Part model, mm, in its own coordinate system. A direction names the side the tool comes from. Give positions to 0.01 mm unless a question says otherwise; leave off trailing zeros. Order: outer loops, then holes, each group sorted by start corner. A loop starts at its lowest first (then second) coordinate and runs counter-clockwise, first axis right, second up. Notation, with made-up numbers: (47, 5.5) - (71, 5.5) arc R25 ccw to (71, 29.5) - close; hole circle Ø3 at (34.25, 85.5). An arc over 180 degrees is marked (long way). Use one line per item in the form item = value. Start each with the question number.
1. Band-saw the part on A-A, the plane z = -35.5. List the corners of the cut face in (x, y) (3 decimals), plus the area to 3 significant figures.
2. Band-saw the part on B-B, the plane y = -7. List the corners of the cut face in (x, z) (3 decimals).
3. Pin check, flat tips, straight feed: P1, Ø3, axis at x = 7, z = -28, coming from the -Y side; P2, Ø1.8, axis at x = 10.325, y = -10.25, coming from the -Z side; P3, Ø6, axis at y = 7.5, z = -42.5, coming from the -X side (3 decimals). Stop position of each tip, or through.
4. Drill centre lines: line 1 (Y direction, x = -12, z = -44); line 2 (Y direction, x = -7, z = -17.5); line 3 (Z direction, x = -8.75, y = 11). Where is each one in solid material? Low to high.
5. Tool access for faces 5 (the face through (10.3, -10.2, 6)), 6 (the face through (12.425, 0, 2)), 7 (the face through (-10.617, 11.744, 5.165)), 8 (the face through (14, -13, -48)): list every direction of +Z, -Z, +X, -X, +Y, -Y with a clear straight run to the whole face (end or side of a thin tool).
6. Pull direction Y, two halves, no side cores. Call faces 1 (the face through (14, 7, -49)), 2 (the face through (-10, -3.5, 2)), 3 (the face through (15, -16.5, -9)), 4 (the face through (-6.85, -13.54, 3.77)): +Y half, -Y half, draft (parallel to the pull), parting line (faces both ways), or undercut.
7. Band-saw the part on C-C, the plane y = 15.5. List the corners of the cut face in (x, z) (3 decimals).
from build123d import *

# Parameters (mm, degrees)
SKETCH2_W           = 33.15
SKETCH2_H           = 33
BOSS_EXTRUDE1_DEPTH = 7.5
SKETCH3_R           = 0.762
CUT_EXTRUDE1_DEPTH  = 6
SKETCH4_W           = 5.3
SKETCH4_H           = 7
CUT_EXTRUDE2_DEPTH  = 3.4
SKETCH5_W           = 17.312690108
SKETCH5_H           = 1.808425299
CUT_EXTRUDE3_DEPTH  = 2
SKETCH6_W           = 5.3
SKETCH6_H           = 3.3
CUT_EXTRUDE4_DEPTH  = 25.560753755
CHAMFER3_SIZE       = 11
CHAMFER3_SIZE2      = 5.848803748
BOSS_EXTRUDE2_DEPTH = 52.5
SKETCH8_W           = 33.15
SKETCH8_H           = 60
BOSS_EXTRUDE3_DEPTH = 1
SKETCH9_W           = 3
SKETCH9_H           = 34
CUT_EXTRUDE5_DEPTH  = 60
SKETCH10_R          = 0.762
CUT_EXTRUDE6_DEPTH  = 6
SKETCH11_R          = 0.762
CUT_EXTRUDE7_DEPTH  = 6
SKETCH12_R          = 0.762
CUT_EXTRUDE9_DEPTH  = 7
SKETCH13_W          = 3
SKETCH13_H          = 5
CUT_EXTRUDE10_DEPTH = 1.5
SKETCH14_W          = 52.5
SKETCH14_H          = 1
BOSS_EXTRUDE4_DEPTH = 1
SKETCH15_R          = 0.762
CUT_EXTRUDE11_DEPTH = 3.5


with BuildPart() as part:
    # Sketch2 → Boss-Extrude1 (new body)
    with BuildSketch(Plane.XY):
        Rectangle(SKETCH2_W, SKETCH2_H)
    extrude(amount=BOSS_EXTRUDE1_DEPTH)

    # Sketch3 → Cut-Extrude1 (cut)
    with BuildSketch(Plane.XY):
        with Locations((10.325, 10.25)):
            Circle(SKETCH3_R)
        with Locations((-10.325, 10.25)):
            Circle(SKETCH3_R)
        with Locations((10.325, -10.25)):
            Circle(SKETCH3_R)
        with Locations((-10.325, -10.25)):
            Circle(SKETCH3_R)
    extrude(amount=CUT_EXTRUDE1_DEPTH, mode=Mode.SUBTRACT)

    # Sketch4 → Cut-Extrude2 (cut)
    with BuildSketch(Plane.XY):
        with Locations((9.775, 0)):
            Rectangle(SKETCH4_W, SKETCH4_H)
        with Locations((-9.775, 0)):
            Rectangle(SKETCH4_W, SKETCH4_H)
    extrude(amount=CUT_EXTRUDE2_DEPTH, mode=Mode.SUBTRACT)

    # Sketch5 → Cut-Extrude3 (cut)
    with BuildSketch(Plane.XY):
        with Locations((-0.109621432, -11.80915301)):
            Rectangle(SKETCH5_W, SKETCH5_H)
    extrude(amount=CUT_EXTRUDE3_DEPTH, mode=Mode.SUBTRACT)

    # Sketch6 → Cut-Extrude4 (cut, through all)
    with BuildSketch(Plane.XY):
        Rectangle(SKETCH6_W, SKETCH6_H)
    extrude(amount=CUT_EXTRUDE4_DEPTH, mode=Mode.SUBTRACT)

    # Chamfer3
    chamfer3_edges = [part.edges().sort_by_distance(p)[0] for p in [
        (2.65, 0, 7.5),
        (0, 1.65, 7.5),
        (-2.65, 0, 7.5),
        (0, -1.65, 7.5),
    ]]
    chamfer3_side = [part.faces().sort_by_distance(p)[0] for p in [
        (-16.107247662, 0, 7.5),
    ]]
    chamfer(chamfer3_edges, length=CHAMFER3_SIZE, length2=CHAMFER3_SIZE2, reference=chamfer3_side[0])

    # Sketch7 → Boss-Extrude2 (add)
    with BuildSketch(Plane.XY):
        Polygon((13.575, -16.5), (17.575, -16.5), (17.575, 16.5), (-16.575, 16.5), (-16.575, -16.5), (-13.575, -16.5), (-13.575, 13.5), (13.575, 13.5), align=None)
    extrude(amount=-BOSS_EXTRUDE2_DEPTH)

    # Sketch8 → Boss-Extrude3 (add)
    with BuildSketch(Plane(origin=(0, 16.5, 0), x_dir=(1, 0, 0), z_dir=(0, 1, 0))):
        with Locations((0, 22.5)):
            Rectangle(SKETCH8_W, SKETCH8_H)
    extrude(amount=BOSS_EXTRUDE3_DEPTH)

    # Sketch9 → Cut-Extrude5 (cut)
    with BuildSketch(Plane(origin=(0, 0, -52.5), x_dir=(-1, 0, 0), z_dir=(0, 0, -1))):
        with Locations((15.075, 0.5)):
            Rectangle(SKETCH9_W, SKETCH9_H)
    extrude(amount=-CUT_EXTRUDE5_DEPTH, mode=Mode.SUBTRACT)

    # Sketch10 → Cut-Extrude6 (cut)
    with BuildSketch(Plane.ZY.offset(13.575)):
        with Locations((-44, 15.5)):
            Circle(SKETCH10_R)
        with Locations(Location((5, 11, 0), (0, 0, 180))):
            Circle(SKETCH10_R)
        with Locations((5, -10)):
            Circle(SKETCH10_R)
    extrude(amount=-CUT_EXTRUDE6_DEPTH, mode=Mode.SUBTRACT)

    # Sketch11 → Cut-Extrude7 (cut)
    with BuildSketch(Plane(origin=(0, -16.5, 0), x_dir=(-1, 0, 0), z_dir=(0, -1, 0))):
        with Locations(Location((-15.575, 44, 0), (0, 0, 90))):
            Circle(SKETCH11_R)
        with Locations((-15.575, -51.5)):
            Circle(SKETCH11_R)
        with Locations(Location((7.075, -4.5, 0), (0, 0, 90))):
            Circle(SKETCH11_R)
        with Locations(Location((-11.075, -4.5, 0), (0, 0, 90))):
            Circle(SKETCH11_R)
    extrude(amount=-CUT_EXTRUDE7_DEPTH, mode=Mode.SUBTRACT)

    # Sketch12 → Cut-Extrude9 (cut)
    with BuildSketch(Plane(origin=(0, 0, -52.5), x_dir=(-1, 0, 0), z_dir=(0, 0, -1))):
        with Locations((-15.575, 15.5)):
            Circle(SKETCH12_R)
        with Locations((-15.575, -14.5)):
            Circle(SKETCH12_R)
        with Locations((11.575, 15.5)):
            Circle(SKETCH12_R)
    extrude(amount=-CUT_EXTRUDE9_DEPTH, mode=Mode.SUBTRACT)

    # Sketch13 → Cut-Extrude10 (cut)
    with BuildSketch(Plane.ZY.offset(-13.575)):
        Polygon((-46.5, 7), (-52.5, 7), (-52.5, -13), (-46.5, -13), (-46.5, -8), align=None)
        with Locations((-45, -10.5)):
            Rectangle(SKETCH13_W, SKETCH13_H)
    extrude(amount=-CUT_EXTRUDE10_DEPTH, mode=Mode.SUBTRACT)

    # Sketch14 → Boss-Extrude4 (add)
    with BuildSketch(Plane(origin=(16.575, 0, 0), x_dir=(0, 0, -1), z_dir=(1, 0, 0))):
        Polygon((0, 17.5), (-7.5, 17.5), (-7.5, -16.5), (0, -16.5), (0, 16.5), align=None)
        with Locations((26.25, 17)):
            Rectangle(SKETCH14_W, SKETCH14_H)
    extrude(amount=BOSS_EXTRUDE4_DEPTH)

    # Sketch15 → Cut-Extrude11 (cut)
    with BuildSketch(Plane.XZ.offset(-13.5)):
        with Locations(Location((-10.813, -7.538, 0), (0, 0, 270))):
            Circle(SKETCH15_R)
        with Locations(Location((10.677, -22.458, 0), (0, 0, 270))):
            Circle(SKETCH15_R)
    extrude(amount=-CUT_EXTRUDE11_DEPTH, mode=Mode.SUBTRACT)


solid = part.part
From the geometry:
q1.outline = (-13.575, 13.5) - (13.575, 13.5) - (13.575, -16.5) - (17.575, -16.5) - (17.575, 17.5) - (-13.575, 17.5) - close
q1.area = 245 mm²
q2.outline = (-13.575, 0) - (13.575, 0) - (13.575, -46.5) - (15.075, -46.5) - (15.075, -52.5) - (17.575, -52.5) - (17.575, 7.5) - (13.65, 7.5) - (8, 4.496) - (-8, 4.496) - (-13.575, 7.46) - close
q3.P1 = 13.5
q3.P2 = 0
q3.P3 = 13.575
q4.line_1 = 13.5 to 14.74, 16.26 to 17.5
q4.line_2 = 13.5 to 17.5
q4.line_3 = 0 to 4.24, 5.76 to 6.62
q5.face_5 = none
q5.face_6 = -Z
q5.face_7 = -X
q5.face_8 = -Z, -X
q6.face_1 = undercut
q6.face_2 = undercut
q6.face_3 = -Y half
q6.face_4 = draft
q7.outline = (-13.575, -52.5) - (-12.337, -52.5) - (-12.337, -45.5) - (-10.813, -45.5) - (-10.813, -52.5) - (14.813, -52.5) - (14.813, -45.5) - (16.337, -45.5) - (16.337, -52.5) - (17.575, -52.5) - (17.575, 7.5) - (-13.575, 7.5) - (-13.575, -43.238) - (-7.575, -43.238) - (-7.575, -44.762) - (-13.575, -44.762) - close; hole circle Ø1.524 at (-10.813, -7.538); hole circle Ø1.524 at (10.677, -22.458)
